Part print with two shaded views. Sizes in mm from the minimum x, y, z corner. A direction names the side the tool comes from. Coordinates: 2 decimals unless noted, no trailing zeros. Order: outer loops, then holes, each group sorted by start corner. A loop starts at its lowest first (then second) coordinate and runs counter-clockwise, first axis right, second up. Notation, with made-up numbers: (45, 70) - (57, 70) arc R23 ccw to (57, 103) - close; hole circle Ø4 at (74, -10.75). An arc over 180 degrees is marked (long way). Write each question's results on one line, items separated by ' | '. Start each with the question number.
Q1. Band-saw the part on C-C, the plane z = 2. Count the separate pieces of the cut face and the enclosed holes in it, then the cut area to 3 significant figures.
Q2. Wall check: probe 1 along Z at (x, y) = (16, 0.8); probe 2 along X at (y, z) = (9.25, 0.55); probe 3 along Y at (x, z) = (10.75, 0.2). Give the ranges that are in metal, low to high.
Q3. Pull direction X, two halves, no side cores. Call the marked faces 5, 6, 7 and 8: released by +X, released by -X, zero draft, split by the parting line, or undercut.
Q4. Pin check, flat tips, straight feed: P1, Ø1.8, axis at x = 16, z = 2, coming from the +Y side; P2, Ø2, axis at x = 18, z = 1.5, coming from the +Y side; P3, Ø5, axis at x = 8, y = 4, coming from the -Z side; P4, Ø1, axis at y = 10, z = 1.5, coming from the -X side. Stop position of each tip, or through.
Q5. Band-saw the part on A-A, the plane y = 5. Write the cut outline in (x, z), then the cut area to 3 significant figures.
Q6. Which spindle directions (+Z, -Z, +X, -X, +Y, -Y) get a long thin tool onto all of the face, cutting with end or side? Do the marked faces 1, 2, 3 and 4. Say none if no direction does.
Q7. Band-saw the part on D-D, the plane x = 11. Write the cut outline in (y, z).
Q8. Band-saw the part on B-B, the plane x = 4. Write the cut outline in (y, z).
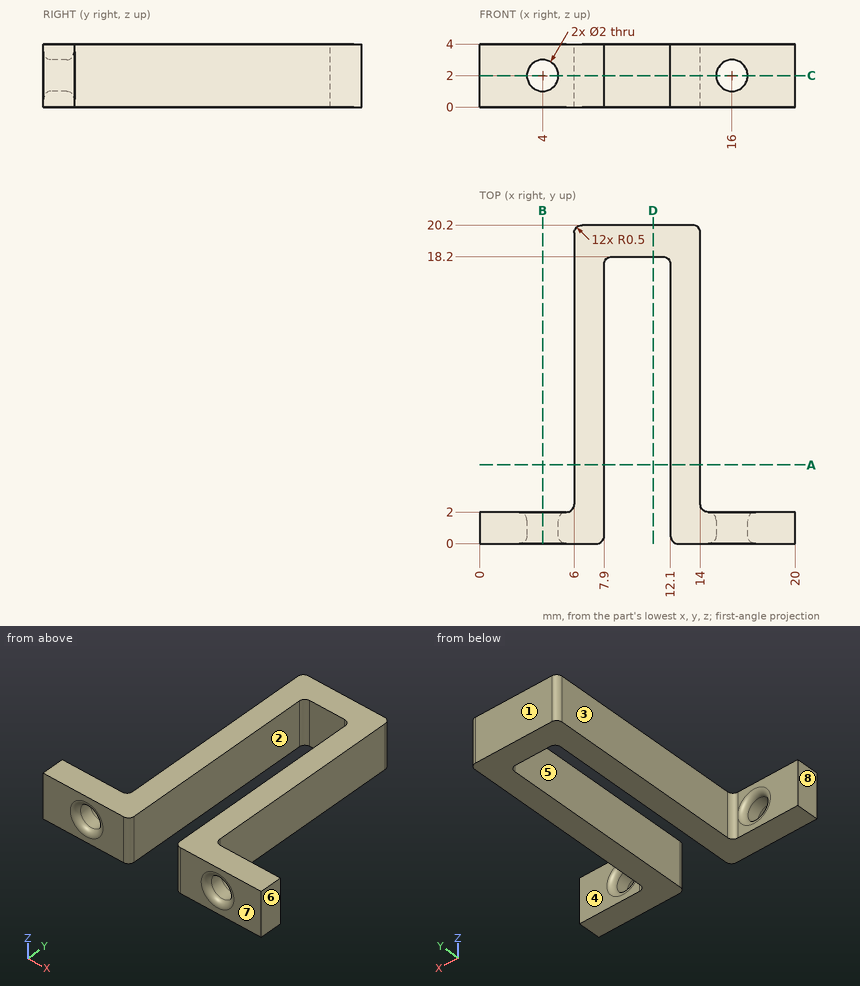
Results below:
1) separate pieces: 3 | enclosed holes: 0 | area: 101 mm²
2) probe 1: z = 0 to 1, 3 to 4 | probe 2: x = 6 to 7.9, 12.1 to 14 | probe 3: y = 18.2 to 20.2
3) face 5: undercut | face 6: released by +X | face 7: zero draft | face 8: released by -X
4) P1: passes through | P2: stops at y = 2 | P3: stops at z = 0 | P4: stops at x = 6
5) outline: (6, 0) - (7.9, 0) - (7.9, 4) - (6, 4) - close; (12.1, 0) - (14, 0) - (14, 4) - (12.1, 4) - close | area: 15.2 mm²
6) face 1: +Z, -Z, +X, -X, +Y | face 2: +Z, -Z, -Y | face 3: +Z, -Z, -X, +Y | face 4: +Z, -Z, +X, +Y
7) outline: (18.2, 0) - (20.2, 0) - (20.2, 4) - (18.2, 4) - close
8) outline: (0, 0) - (2, 0) - (2, 0.5) arc R0.5 ccw to (1.5, 1) - (0.5, 1) arc R0.5 ccw to (0, 0.5) - close; (0, 3.5) arc R0.5 ccw to (0.5, 3) - (1.5, 3) arc R0.5 ccw to (2, 3.5) - (2, 4) - (0, 4) - close
